Design review of the part built by this model. Coordinates are the model's own, in mm. A direction names the side the tool comes from. Coordinates: 2 decimals unless noted, no trailing zeros. Order: outer loops, then holes, each group sorted by start corner. A loop starts at its lowest first (then second) coordinate and runs counter-clockwise, first axis right, second up. Notation, with made-up numbers: M -26.75,11.25 L 8.25,11.25 A37 cw 8.25,48.25 Z; hole C 82.25,53.25 d11. An arc over 180 degrees is marked long. Answer in a Markdown table with one row per item.
from build123d import *

# Parameters (mm, degrees)
BOSS_EXTRUDE1_DEPTH               = 20
TAP_DRILL_FOR_M3_TAP1_D           = 2.5
TAP_DRILL_FOR_M3_TAP1_CSINK_D     = 2.8
TAP_DRILL_FOR_M3_TAP1_CSINK_ANGLE = 90
TAP_DRILL_FOR_M4_TAP1_D           = 3.3
TAP_DRILL_FOR_M4_TAP1_CSINK_D     = 3.35
TAP_DRILL_FOR_M4_TAP1_CSINK_ANGLE = 90


with BuildPart() as part:
    # Sketch1 → Boss-Extrude1 (new body)
    with BuildSketch(Plane.XY):
        Polygon((5.74072013, -5), (27.5, -5), (27.5, 5), (-27.5, 5), (-27.5, -5), (-5.74072013, -5), (-5.74072013, -25), (5.74072013, -25), align=None)
    extrude(amount=BOSS_EXTRUDE1_DEPTH)

    # Tap Drill for M3 Tap1 (through all)
    with Locations(Plane(origin=(0, -8.9, 20), x_dir=(1, 0, 0), z_dir=(0, 0, 1))):
        with Locations((0, 0)):
            CounterSinkHole(TAP_DRILL_FOR_M3_TAP1_D / 2, TAP_DRILL_FOR_M3_TAP1_CSINK_D / 2, counter_sink_angle=TAP_DRILL_FOR_M3_TAP1_CSINK_ANGLE)

    # Tap Drill for M4 Tap1 (through all)
    with Locations(Plane(origin=(13.78, -5, 10), x_dir=(0, 0, -1), z_dir=(0, -1, 0))):
        with Locations((0, 0), (0, -27.5)):
            CounterSinkHole(TAP_DRILL_FOR_M4_TAP1_D / 2, TAP_DRILL_FOR_M4_TAP1_CSINK_D / 2, counter_sink_angle=TAP_DRILL_FOR_M4_TAP1_CSINK_ANGLE)


solid = part.part
(1) Add section D-D, the plane z = 6. Give the boundary of the cut face in (x, y), and give its area (3 significant figures).
Return value:
| item | result |
|---|---|
| outline | M -27.5,-5 L -5.74,-5 L -5.74,-25 L 5.74,-25 L 5.74,-5 L 27.5,-5 L 27.5,5 L -27.5,5 Z; hole C 0,-8.9 d2.5 |
| area | 775 mm2 |
(2) For line 1 along X through (y, z) = (0, 10); line 2 along X through (y, z) = (-8.9, 12.75); line 3 along Z through (x, y) = (-13.72, -2.25), list the stretches that pass through material, from the lowest coordinate up. Write a range as from..to.
Return value:
| item | result |
|---|---|
| line 1 | x = -27.5..-15.37, -12.07..12.13, 15.43..27.5 |
| line 2 | x = -5.74..-1.25, 1.25..5.74 |
| line 3 | z = 0..8.35, 11.65..20 |
(3) Add section A-A, the plane z = 10. Give the boundary of the cut face in (x, y) (3 decimals).
Return value:
| item | result |
|---|---|
| outline | M -27.5,-5 L -15.395,-5 L -15.37,-4.975 L -15.37,5 L -27.5,5 Z; M -12.07,-4.975 L -12.045,-5 L -5.741,-5 L -5.741,-25 L 5.741,-25 L 5.741,-5 L 12.105,-5 L 12.13,-4.975 L 12.13,5 L -12.07,5 Z; M 15.43,-4.975 L 15.455,-5 L 27.5,-5 L 27.5,5 L 15.43,5 Z; hole C 0,-8.9 d2.5 |
(4) Draft analysis for pull direction Y (two halves, no side actions). For faces 1 (the cylindrical face through (-0.577, -10.009, 9.786)), 2 (the flat face through (0, -3, 20)), 3 (the flat face through (-17, -5, 10)), state which applies: pulls with the +Y half, pulls with the -Y half, needs draft (parallel to the pull), parting line crosses it, or undercut.
Return value:
| item | result |
|---|---|
| face 1 | undercut |
| face 2 | needs draft |
| face 3 | pulls with the -Y half |
(5) Insertion check: pin 1 Ø4 at (y, z) = (-9.5, 5.5) entering from +X; pin 2 Ø4.5 at (x, z) = (13.78, 10) entering from -Y. Each pin has a flat end and moves straight along its axis. Give the tip position at first contact, or say it passes through.
Return value:
| item | result |
|---|---|
| pin 1 | stops at x = 5.74 |
| pin 2 | stops at y = -5 |
(6) Add section C-C, the plane y = 3. Give the boundary of the cut face in (x, z), and give its area (3 significant figures).
Return value:
| item | result |
|---|---|
| outline | M -27.5,0 L 27.5,0 L 27.5,20 L -27.5,20 Z; hole C -13.72,10 d3.3; hole C 13.78,10 d3.3 |
| area | 1,080 mm2 |
(7) Add section B-B, the plane x = -13.72. Give the boundary of the cut face in (y, z) (3 decimals).
Return value:
| item | result |
|---|---|
| outline | M -5,0 L 5,0 L 5,8.35 L -4.975,8.35 L -5,8.325 Z; M -5,11.675 L -4.975,11.65 L 5,11.65 L 5,20 L -5,20 Z |
(8) For faces 4 (the flat face through (0, -3, 0)), 5 (the flat face through (-5.741, -15, 10)), 6 (the flat face through (5.741, -15, 10)), list the 3-axis set-ups (+Z, -Z, +X, -X, +Y, -Y) from which the entire face can be reached by the end or side of a thin tool; tool diameter is ignored.
Return value:
| item | result |
|---|---|
| face 4 | -Z, +X, -X, +Y, -Y |
| face 5 | +Z, -Z, -X, -Y |
| face 6 | +Z, -Z, +X, -Y |
